Input: part model. Units: mm. Frame: model coordinates. Give positions to 0.01 mm unless a question says otherwise; leave off trailing zeros. Order: outer loops, then holes, each group sorted by start corner. A loop starts at its lowest first (then second) coordinate and runs counter-clockwise, first axis right, second up. Notation, with made-up numbers: M -8.75,-4.75 L 46.25,-4.75 A15 ccw 46.25,21.25 Z; hole C -16,28 d3. An arc over 180 degrees is marked long. Use a Markdown table: item, result.
from build123d import *

# Parameters (mm, degrees)
BOSS_EXTRUDE1_DEPTH = 19.05
SKETCH2_W           = 119.77527386
SKETCH2_H           = 145.609156457
CUT_EXTRUDE1_DEPTH  = 25.4
SKETCH3_R           = 101.6
CUT_EXTRUDE2_DEPTH  = 85.36695047


with BuildPart() as part:
    # Sketch1 → Boss-Extrude1 (new body)
    with BuildSketch(Plane.XY):
        Polygon((-78.164696837, 0), (-63.5, 25.4), (63.5, 25.4), (78.164696837, 0), align=None)
    extrude(amount=-BOSS_EXTRUDE1_DEPTH)

    # Sketch2 → Cut-Extrude1 (cut)
    with BuildSketch(Plane(origin=(58.623522628, 33.84630657, 0), x_dir=(0, 0, -1), z_dir=(0.866025403784436, 0.5000000000000047, 0))):
        with Locations((20.492508396, -22.352934086)):
            Rectangle(SKETCH2_W, SKETCH2_H)
    extrude(amount=-CUT_EXTRUDE1_DEPTH, mode=Mode.SUBTRACT)

    # Sketch3 → Cut-Extrude2 (cut, through all)
    with BuildSketch(Plane.XY):
        with Locations((-14.664696837, -84.31457873)):
            Circle(SKETCH3_R)
    extrude(amount=-CUT_EXTRUDE2_DEPTH, mode=Mode.SUBTRACT)


solid = part.part
1) First-contact query: pin 1 Ø5 at (y, z) = (18.5, -16) entering from +X; pin 2 Ø1 at (y, z) = (12, -17) entering from +X; pin 3 Ø3 at (x, z) = (-2.5, -14.5) entering from -Y; pin 4 Ø8 at (x, y) = (-13, 14.5) entering from +Z. Flat tips, straight axial feed; report the tip coordinate or a pass-through.
Response values:
| item | result |
|---|---|
| pin 1 | stops at x = 39.6 |
| pin 2 | stops at x = 42.2 |
| pin 3 | stops at y = 16.36 |
| pin 4 | stops at z = 0 |
2) Cut plane A-A on y = 10.5. Return loops of the section in (x, z), and give its area (3 significant figures).
Response values:
| item | result |
|---|---|
| outline | M -72.1,-19.05 L -51.17,-19.05 L -51.17,0 L -72.1,0 Z; M 21.84,-19.05 L 42.77,-19.05 L 42.77,0 L 21.84,0 Z |
| area | 797 mm² |
3) Material intervals for line 1 (X direction, y = 5.5, z = -2.25); line 2 (X direction, y = 6, z = -16.25); line 3 (X direction, y = 20, z = -6.5), sorted ascending. Write a range as from..to.
Response values:
| item | result |
|---|---|
| line 1 | x = -74.99..-62.16, 32.83..45.66 |
| line 2 | x = -74.7..-61.2, 31.87..45.37 |
| line 3 | x = -66.62..37.29 |
4) Cut plane C-C on y = 1.75. Return loops of the section in (x, z), and give its area (3 significant figures).
Response values:
| item | result |
|---|---|
| outline | M -77.15,-19.05 L -68.66,-19.05 L -68.66,0 L -77.15,0 Z; M 39.33,-19.05 L 47.82,-19.05 L 47.82,0 L 39.33,0 Z |
| area | 324 mm² |
5) Mould query, pull axis X, two halves, no side actions, for faces 1 (the face through (-14, 19, 0)), 2 (the face through (-13.82, 17.28, -9.39)), 3 (the face through (-70.935, 12.522, -9.392)). Classes: released by +X, released by -X, zero draft, split by the parting line, or undercut.
Response values:
| item | result |
|---|---|
| face 1 | zero draft |
| face 2 | undercut |
| face 3 | released by -X |
6) Cut plane D-D on x = 17. Return loops of the section in (y, z), and give its area (3 significant figures).
Response values:
| item | result |
|---|---|
| outline | M 12.23,-19.05 L 25.4,-19.05 L 25.4,0 L 12.23,0 Z |
| area | 251 mm² |
7) Cut plane B-B on z = -4.5. Return loops of the section in (x, y).
Response values:
| item | result |
|---|---|
| outline | M -78.16,0 L -71.35,0 A101.6 cw 42.02,0 L 48.84,0 L 34.17,25.4 L -63.5,25.4 Z |
